Can you work these out from the model? Positions are in its coordinate system, mm. A direction names the side the tool comes from. Give positions to 0.01 mm unless a question says otherwise; leave off trailing zeros. Return JSON: item names as keys, results as strings. Group by question number.
from build123d import *

# Parameters (mm, degrees)
SKETCH_1_W                  = 340
SKETCH_1_H                  = 450
EXTRUDE_1_DEPTH             = 12
HOLE_WIZARD_3_D             = 6.6
HOLE_WIZARD_3_CBORE_D       = 11
HOLE_WIZARD_3_CBORE_DEPTH   = 6.8
HOLE_WIZARD_3_2_D           = 4.5
HOLE_WIZARD_3_2_CBORE_D     = 8
HOLE_WIZARD_3_2_CBORE_DEPTH = 4.6
HOLE_WIZARD_M6_1_D          = 5
HOLE_WIZARD_1_D             = 18
HOLE_WIZARD_1_DEPTH         = 2
CUT_EXTRUDE_1_DEPTH         = 283.256975113
CHAMFER_1_SIZE              = 2


with BuildPart() as part:
    # 草图1 → 凸台-拉伸1 (new body)
    with BuildSketch(Plane(origin=(0, 0, 0), x_dir=(1, 0, 0), z_dir=(0, 1, 0))):
        Rectangle(SKETCH_1_W, SKETCH_1_H)
    extrude(amount=EXTRUDE_1_DEPTH)

    # Hole Wizard 3 (through all)
    with Locations(Plane(origin=(0, 12, 0), x_dir=(1, 0, 0), z_dir=(0, 1, 0))):
        with Locations((-115, 65), (-115, 105), (-155, 105), (-155, 65), (155, 65), (155, 105), (115, 105), (115, 65), (115, -65), (115, -105), (155, -105), (155, -65), (-155, -65), (-155, -105), (-115, -105), (-115, -65)):
            CounterBoreHole(HOLE_WIZARD_3_D / 2, HOLE_WIZARD_3_CBORE_D / 2, HOLE_WIZARD_3_CBORE_DEPTH)

    # Hole Wizard 3 2 (through all)
    with Locations(Plane(origin=(0, 12, 0), x_dir=(1, 0, 0), z_dir=(0, 1, 0))):
        with Locations((20, 7.5), (20, -7.5), (-6.7, 25), (-6.7, 35)):
            CounterBoreHole(HOLE_WIZARD_3_2_D / 2, HOLE_WIZARD_3_2_CBORE_D / 2, HOLE_WIZARD_3_2_CBORE_DEPTH)

    # M6 螺纹孔1 (through all)
    with Locations(Plane(origin=(-174.714463093, 0, 28.629345755), x_dir=(1, 0, 0), z_dir=(0, -1, 0))):
        with Locations((19.714463093, -236.129345755), (19.714463093, -46.129345755), (329.714463093, -46.129345755), (329.714463093, -236.129345755), (329.714463093, 178.870654245), (329.714463093, -11.129345755), (19.714463093, -11.129345755), (19.714463093, 178.870654245)):
            Hole(HOLE_WIZARD_M6_1_D / 2)

    # 孔1
    with Locations(Plane(origin=(0, 12, 0), x_dir=(1, 0, 0), z_dir=(0, 1, 0))):
        with Locations((-155, 17.5), (-155, 207.5), (155, 207.5), (155, 17.5), (155, -17.5), (155, -207.5), (-155, -207.5), (-155, -17.5)):
            Hole(HOLE_WIZARD_1_D / 2, depth=HOLE_WIZARD_1_DEPTH)

    # 草图13 → 切除-拉伸1 (cut, through all)
    with BuildSketch(Plane(origin=(0, 12, 0), x_dir=(1, 0, 0), z_dir=(0, 1, 0))):
        with BuildLine():
            Line((-167, 62.5), (-170, 62.5))
            Line((-170, 62.5), (-170, 162.5))
            Line((-170, 162.5), (-147, 162.5))
            ThreePointArc((-147, 162.5), (-143.464466094, 161.035533906), (-142, 157.5))
            Line((-142, 157.5), (-142, 117))
            ThreePointArc((-142, 117), (-143.464466094, 113.464466094), (-147, 112))
            Line((-147, 112), (-162, 112))
            Line((-162, 112), (-162, 67.5))
            ThreePointArc((-162, 67.5), (-163.464466094, 63.964466094), (-167, 62.5))
        make_face()
        with BuildLine():
            Line((142, 117), (142, 157.5))
            ThreePointArc((142, 157.5), (143.464466094, 161.035533906), (147, 162.5))
            Line((147, 162.5), (170, 162.5))
            Line((170, 162.5), (170, 62.5))
            Line((170, 62.5), (167, 62.5))
            ThreePointArc((167, 62.5), (163.464466094, 63.964466094), (162, 67.5))
            Line((162, 67.5), (162, 112))
            Line((162, 112), (147, 112))
            ThreePointArc((147, 112), (143.464466094, 113.464466094), (142, 117))
        make_face()
        with BuildLine():
            Line((-142, -117), (-142, -157.5))
            ThreePointArc((-142, -157.5), (-143.464466094, -161.035533906), (-147, -162.5))
            Line((-147, -162.5), (-170, -162.5))
            Line((-170, -162.5), (-170, -62.5))
            Line((-170, -62.5), (-167, -62.5))
            ThreePointArc((-167, -62.5), (-163.464466094, -63.964466094), (-162, -67.5))
            Line((-162, -67.5), (-162, -112))
            Line((-162, -112), (-147, -112))
            ThreePointArc((-147, -112), (-143.464466094, -113.464466094), (-142, -117))
        make_face()
        with BuildLine():
            Line((167, -62.5), (170, -62.5))
            Line((170, -62.5), (170, -162.5))
            Line((170, -162.5), (147, -162.5))
            ThreePointArc((147, -162.5), (143.464466094, -161.035533906), (142, -157.5))
            Line((142, -157.5), (142, -117))
            ThreePointArc((142, -117), (143.464466094, -113.464466094), (147, -112))
            Line((147, -112), (162, -112))
            Line((162, -112), (162, -67.5))
            ThreePointArc((162, -67.5), (163.464466094, -63.964466094), (167, -62.5))
        make_face()
    extrude(amount=-CUT_EXTRUDE_1_DEPTH, mode=Mode.SUBTRACT)

    # 倒角1
    chamfer_1_edges = [part.edges().sort_by_distance(p)[0] for p in [
        (-170, 6, -62.5),
        (-170, 6, -162.5),
        (-162, 6, -112),
        (170, 6, -62.5),
        (162, 6, -112),
        (170, 6, -162.5),
        (170, 6, 62.5),
        (170, 6, 162.5),
        (162, 6, 112),
        (-170, 6, 62.5),
        (-162, 6, 112),
        (170, 6, 225),
        (-170, 6, 225),
        (-170, 6, -225),
        (170, 6, -225),
    ]]
    chamfer(chamfer_1_edges, length=CHAMFER_1_SIZE)


solid = part.part
1) Imagine slicing it at A-A, the plane y = 2.5. Count the separate pieces of the cut face and the enclosed holes in it, and give its area (3 significant figures).
2) I need wall thicknesses on line 1 along X through (y, z) = (9.5, -105); line 2 along Z through (x, y) = (-115, 9.75); line 3 along Z through (x, y) = (115, 1.6). Which ranges of each line are inside material? Lowest first, please.
3) On a 3-axis mill with a long thin cutter (end or side, diameter ignored), from which of +Z, -Z, +X, -X, +Y, -Y can I reach the whole of each face in a straight line? I mean faces 1 (the face through (115, 5.2, -61)), 2 (the face through (162, 6, -88)), 3 (the face through (-142, 6, 137)). Say none if no direction works.
4) We'd pull the mould along Z, two halves only. Please class faces 4 (the face through (-153.828, 10.986, -216.423)), 5 (the face through (170, 6, 194)), 6 (the face through (-2, 6, 225)), 7 (the face through (163.99, 10.99, -17.9)): pulls with the +Z half, pulls with the -Z half, needs draft (parallel to the pull), parting line crosses it, or undercut.
5) Will these pins go through, and if not, where does the flat tip stop? pin 1 Ø3 at (y, z) = (8, 124) entering from -X; pin 2 Ø5.5 at (x, z) = (-158, -210.5) entering from +Y; pin 3 Ø3.5 at (x, z) = (-116, 107) entering from +Y; pin 4 Ø5.5 at (x, z) = (115, 105) entering from +Y.
Resolved:
{
 "1": {"separate pieces": "1", "enclosed holes": "28", "area": "145,000 mm^2"},
 "2": {"line 1": "-162 to -160.5, -149.5 to -120.5, -109.5 to 109.5, 120.5 to 149.5, 160.5 to 162", "line 2": "-225 to -110.5, -99.5 to -70.5, -59.5 to 59.5, 70.5 to 99.5, 110.5 to 225", "line 3": "-225 to -108.3, -101.7 to -68.3, -61.7 to 61.7, 68.3 to 101.7, 108.3 to 225"},
 "3": {"face 1": "+Y", "face 2": "+X, +Y, -Y", "face 3": "-X, +Y, -Y"},
 "4": {"face 4": "undercut", "face 5": "needs draft", "face 6": "pulls with the +Z half", "face 7": "undercut"},
 "5": {"pin 1": "x = -142", "pin 2": "y = 10", "pin 3": "y = 5.2", "pin 4": "through"}
}
